from build123d import *

# Parameters (mm, degrees)
SKETCH2_W           = 42.3
SKETCH2_H           = 42.3
SKETCH2_R           = 1.6
SKETCH2_W_2         = 20
SKETCH2_R_2         = 2.6
BOSS_EXTRUDE1_DEPTH = 5
SKETCH3_R           = 12.5
CUT_EXTRUDE1_DEPTH  = 10


with BuildPart() as part:
    # Sketch2 → Boss-Extrude1 (new body)
    with BuildSketch(Plane.XY):
        Rectangle(SKETCH2_W, SKETCH2_H)
        with Locations((-15.5, -15.5)):
            Circle(SKETCH2_R, mode=Mode.SUBTRACT)
        with Locations((15.5, 15.5)):
            Circle(SKETCH2_R, mode=Mode.SUBTRACT)
        with Locations((15.5, -15.5)):
            Circle(SKETCH2_R, mode=Mode.SUBTRACT)
        with Locations((-15.5, 15.5)):
            Circle(SKETCH2_R, mode=Mode.SUBTRACT)
        with Locations((31.15, 0)):
            Rectangle(SKETCH2_W_2, SKETCH2_H)
        with Locations((31.15, -11.15)):
            Circle(SKETCH2_R_2, mode=Mode.SUBTRACT)
        with Locations((31.15, 11.15)):
            Circle(SKETCH2_R_2, mode=Mode.SUBTRACT)
    extrude(amount=BOSS_EXTRUDE1_DEPTH)

    # Sketch3 → Cut-Extrude1 (cut)
    with BuildSketch(Plane(origin=(0, 0, 0), x_dir=(-1, 0, 0), z_dir=(0, 0, -1))):
        Circle(SKETCH3_R)
    extrude(amount=-CUT_EXTRUDE1_DEPTH, mode=Mode.SUBTRACT)


solid = part.part
Can you work these out from the model? Positions are in its coordinate system, mm. Round coordinates to 2 decimals unless told otherwise and drop trailing zeros. Order: outer loops, then holes, each group sorted by start corner. A loop starts at its lowest first (then second) coordinate and runs counter-clockwise, first axis right, second up. Notation, with made-up numbers: (4.25, -3.5) - (30.25, -3.5) arc R28 cw to (30.25, 27.5) - close; hole circle Ø4 at (13.5, 68.5). An arc over 180 degrees is marked (long way). Answer in a Markdown table with one row per item.
(1) Suppose I cut it at C-C, the plane y = 0. Please give me the cut outline in (x, z).
From the geometry:
| item | result |
|---|---|
| outline | (-21.15, 0) - (-12.5, 0) - (-12.5, 5) - (-21.15, 5) - close; (12.5, 0) - (41.15, 0) - (41.15, 5) - (12.5, 5) - close |
(2) Suppose I cut it at D-D, the plane z = 1.25. Please give me the cut outline in (x, y), plus the area to 3 significant figures.
From the geometry:
| item | result |
|---|---|
| outline | (-21.15, -21.15) - (41.15, -21.15) - (41.15, 21.15) - (-21.15, 21.15) - close; hole circle Ø3.2 at (-15.5, -15.5); hole circle Ø3.2 at (-15.5, 15.5); hole circle Ø25 at (0, 0); hole circle Ø3.2 at (15.5, -15.5); hole circle Ø3.2 at (15.5, 15.5); hole circle Ø5.2 at (31.15, -11.15); hole circle Ø5.2 at (31.15, 11.15) |
| area | 2,070 mm2 |
(3) If we mould it in two halves opening along X, with no side actions, what happens to faces 1 (the face through (10, -21.15, 2)), 2 (the face through (41.15, 0, 2)), 3 (the face through (-16.68, 16.58, 2.46)), 4 (the face through (-21.15, 0, 2))? For each: released by +X, released by -X, zero draft, split by the parting line, or undercut.
From the geometry:
| item | result |
|---|---|
| face 1 | zero draft |
| face 2 | released by +X |
| face 3 | undercut |
| face 4 | released by -X |
(4) Please list where these lines run through material, in increasing order: L1, parallel to Y at x = 31.15, z = 3.25; L2, parallel to Y at x = -15.5, z = 3.45; L3, parallel to X at y = 7, z = 1.25. Write a range as from..to.
From the geometry:
| item | result |
|---|---|
| L1 | y = -21.15..-13.75, -8.55..8.55, 13.75..21.15 |
| L2 | y = -21.15..-17.1, -13.9..13.9, 17.1..21.15 |
| L3 | x = -21.15..-10.36, 10.36..41.15 |
(5) Suppose I cut it at A-A, the plane y = -15.5. Please give me the cut outline in (x, z), plus the area to 4 significant figures.
From the geometry:
| item | result |
|---|---|
| outline | (-21.15, 0) - (-17.1, 0) - (-17.1, 5) - (-21.15, 5) - close; (-13.9, 0) - (13.9, 0) - (13.9, 5) - (-13.9, 5) - close; (17.1, 0) - (41.15, 0) - (41.15, 5) - (17.1, 5) - close |
| area | 279.5 mm2 |
(6) Suppose I cut it at B-B, the plane x = 15.5. Please give me the cut outline in (y, z), plus the area to 4 significant figures.
From the geometry:
| item | result |
|---|---|
| outline | (-21.15, 0) - (-17.1, 0) - (-17.1, 5) - (-21.15, 5) - close; (-13.9, 0) - (13.9, 0) - (13.9, 5) - (-13.9, 5) - close; (17.1, 0) - (21.15, 0) - (21.15, 5) - (17.1, 5) - close |
| area | 179.5 mm2 |
(7) For P1, Ø20, axis at x = 0, y = 0, coming from the +Z side, with a flat end and sliding along its axis, tell me the tip position at first contact or that it passes through.
From the geometry:
| item | result |
|---|---|
| P1 | passes through |
